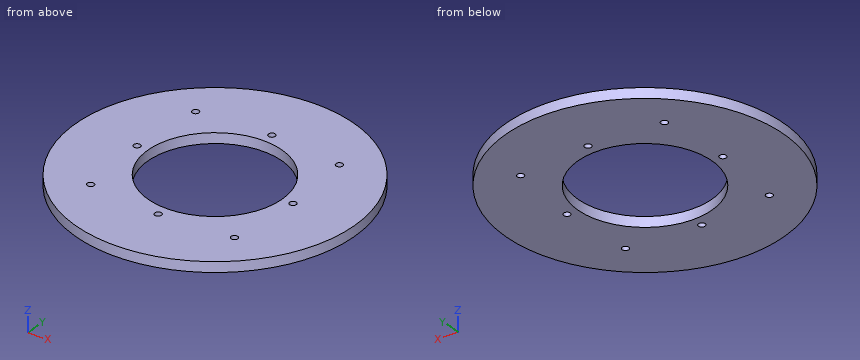
```python
from build123d import *

# Parameters (mm, degrees)
SKETCH1_R           = 82
SKETCH1_R_2         = 39.5
BOSS_EXTRUDE1_DEPTH = 6
SKETCH2_R           = 2
CUT_EXTRUDE1_DEPTH  = 10
CIRPATTERN1_COUNT   = 4
SKETCH3_R           = 2
CUT_EXTRUDE2_DEPTH  = 10


with BuildPart() as part:
    # Sketch1 → Boss-Extrude1 (new body)
    with BuildSketch(Plane.XY):
        Circle(SKETCH1_R)
        Circle(SKETCH1_R_2, mode=Mode.SUBTRACT)
    extrude(amount=BOSS_EXTRUDE1_DEPTH)

    # Sketch2 → Cut-Extrude1 (cut)
    with BuildSketch(Plane.XY.offset(6)):
        with Locations((42.426406871, 42.426406871)):
            Circle(SKETCH2_R)
    cut_extrude1 = extrude(amount=-CUT_EXTRUDE1_DEPTH, mode=Mode.SUBTRACT)

    # CirPattern1: Cut-Extrude1 ×4 about axis
    cirpattern1_axis = Axis((0, 0, 0), (0, 0, 1))
    for i in range(1, CIRPATTERN1_COUNT):
        add(cut_extrude1.rotate(cirpattern1_axis, i * 360 / CIRPATTERN1_COUNT), mode=Mode.SUBTRACT)

    # Sketch3 → Cut-Extrude2 (cut)
    with BuildSketch(Plane.XY.offset(6)):
        with Locations((0, 46)):
            Circle(SKETCH3_R)
        with Locations((46, 0)):
            Circle(SKETCH3_R)
        with Locations((0, -46)):
            Circle(SKETCH3_R)
        with Locations((-46, 0)):
            Circle(SKETCH3_R)
    extrude(amount=-CUT_EXTRUDE2_DEPTH, mode=Mode.SUBTRACT)


solid = part.part
```
Input: part model. Units: mm. Frame: model coordinates. Give positions to 0.01 mm unless a question says otherwise; leave off trailing zeros. Order: outer loops, then holes, each group sorted by start corner. A loop starts at its lowest first (then second) coordinate and runs counter-clockwise, first axis right, second up. Notation, with made-up numbers: (19.25, 25.25) -> (51.25, 25.25) arc R21 ccw to (51.25, 42.25) -> close; hole circle Ø8 at (66.25, 70). An arc over 180 degrees is marked (long way). Write each question's results on one line, items separated by ' | '. Start each with the question number.
Item 1: Contact query for flat-ended pins moving along their axis: P1, Ø3, axis at y = 41.5, z = 2, coming from the +X side; P2, Ø2.5, axis at x = 0, y = -46, coming from the -Z side. Output: stop coordinate, or through.
Item 2: Cut plane A-A on y = 0. Return the cut outline in (x, z).
Item 3: Cut plane C-C on z = 2.65. Give the number of separate pieces and of enclosed holes in the cut face, then the cut area to 3 significant figures.
Item 4: Cut plane D-D on x = -27. Return the cut outline in (y, z), then the cut area to 3 significant figures.
Item 5: Line query: line 1 (Y direction, x = 0, z = 2.5); line 2 (X direction, y = 41.5, z = 3.75); line 3 (Y direction, x = -28.5, z = 2). Output: solid intervals per line, ascending.
Established:
1) P1: x = 71.58 | P2: through
2) outline: (-82, 0) -> (-48, 0) -> (-48, 6) -> (-82, 6) -> close; (-44, 0) -> (-39.5, 0) -> (-39.5, 6) -> (-44, 6) -> close; (39.5, 0) -> (44, 0) -> (44, 6) -> (39.5, 6) -> close; (48, 0) -> (82, 0) -> (82, 6) -> (48, 6) -> close
3) separate pieces: 1 | enclosed holes: 9 | area: 16,100 mm^2
4) outline: (-77.43, 0) -> (-28.83, 0) -> (-28.83, 6) -> (-77.43, 6) -> close; (28.83, 0) -> (77.43, 0) -> (77.43, 6) -> (28.83, 6) -> close | area: 583 mm^2
5) line 1: -82 to -48, -44 to -39.5, 39.5 to 44, 48 to 82 | line 2: -70.72 to -44.2, -40.65 to 40.65, 44.2 to 70.72 | line 3: -76.89 to -27.35, 27.35 to 76.89
